```python
from build123d import *

# Parameters (mm, degrees)
SKETCH1_W           = 25
SKETCH1_H           = 40
BOSS_EXTRUDE1_DEPTH = 50
SKETCH2_R           = 4.1
CUT_EXTRUDE1_DEPTH  = 51
SKETCH3_R           = 4.1
CUT_EXTRUDE2_DEPTH  = 41
CUT_EXTRUDE3_DEPTH  = 21
BOSS_EXTRUDE2_DEPTH = 10
BOSS_EXTRUDE3_DEPTH = 10
CHAMFER1_SIZE       = 1
BOSS_EXTRUDE4_DEPTH = 10


with BuildPart() as part:
    # Sketch1 → Boss-Extrude1 (new body)
    with BuildSketch(Plane(origin=(0, 0, 0), x_dir=(1, 0, 0), z_dir=(0, 1, 0))):
        Rectangle(SKETCH1_W, SKETCH1_H)
    extrude(amount=BOSS_EXTRUDE1_DEPTH)

    # Sketch2 → Cut-Extrude1 (cut, through all)
    with BuildSketch(Plane.XZ):
        with Locations((0, -10)):
            Circle(SKETCH2_R)
    extrude(amount=-CUT_EXTRUDE1_DEPTH, mode=Mode.SUBTRACT)

    # Sketch3 → Cut-Extrude2 (cut, through all)
    with BuildSketch(Plane.XY.offset(20)):
        with Locations((0, 17)):
            Circle(SKETCH3_R)
        with Locations((0, 33)):
            Circle(SKETCH3_R)
    extrude(amount=-CUT_EXTRUDE2_DEPTH, mode=Mode.SUBTRACT)

    # Sketch4 → Cut-Extrude3 (cut)
    with BuildSketch(Plane(origin=(0, 0, -20), x_dir=(-1, 0, 0), z_dir=(0, 0, -1))):
        Polygon((-7.5, 17), (-3.75, 10.504809472), (3.75, 10.504809472), (7.5, 17), (3.75, 23.495190528), (-3.75, 23.495190528), align=None)
        Polygon((3.75, 39.495190528), (-3.75, 39.495190528), (-7.5, 33), (-3.75, 26.504809472), (3.75, 26.504809472), (7.5, 33), align=None)
    extrude(amount=-CUT_EXTRUDE3_DEPTH, mode=Mode.SUBTRACT)

    # Sketch5 → Boss-Extrude2 (add)
    with BuildSketch(Plane(origin=(0, 50, 0), x_dir=(1, 0, 0), z_dir=(0, 1, 0))):
        with BuildLine():
            Line((12.5, 5), (20.5, 5))
            Line((20.5, 5), (20.5, 8.1))
            Line((20.5, 8.1), (18.821637353, 8.1))
            ThreePointArc((18.821637353, 8.1), (13.5, 10), (18.821637353, 11.9))
            Line((18.821637353, 11.9), (20.5, 11.9))
            Line((20.5, 11.9), (20.5, 15))
            Line((20.5, 15), (12.5, 15))
            Line((12.5, 15), (12.5, 5))
        make_face()
    extrude(amount=-BOSS_EXTRUDE2_DEPTH)

    # Sketch6 → Boss-Extrude3 (add)
    with BuildSketch(Plane.XY.offset(20)):
        with BuildLine():
            Line((12.5, 12), (20.5, 12))
            Line((20.5, 12), (20.5, 15.1))
            Line((20.5, 15.1), (18.821637353, 15.1))
            ThreePointArc((18.821637353, 15.1), (13.5, 17), (18.821637353, 18.9))
            Line((18.821637353, 18.9), (20.5, 18.9))
            Line((20.5, 18.9), (20.5, 22))
            Line((20.5, 22), (12.5, 22))
            Line((12.5, 22), (12.5, 12))
        make_face()
    extrude(amount=-BOSS_EXTRUDE3_DEPTH)

    # Chamfer1
    chamfer1_edges = [part.edges().sort_by_distance(p)[0] for p in [
        (5.625, 20.247595264, -20),
        (5.625, 13.752404736, -20),
        (0, 10.504809472, -20),
        (-5.625, 13.752404736, -20),
        (-5.625, 20.247595264, -20),
        (0, 23.495190528, -20),
        (-5.625, 36.247595264, -20),
        (0, 39.495190528, -20),
        (5.625, 36.247595264, -20),
        (5.625, 29.752404736, -20),
        (0, 26.504809472, -20),
        (-5.625, 29.752404736, -20),
    ]]
    chamfer(chamfer1_edges, length=CHAMFER1_SIZE)

    # Sketch7 → Boss-Extrude4 (add)
    with BuildSketch(Plane(origin=(0, 50, 0), x_dir=(1, 0, 0), z_dir=(0, 1, 0))):
        Polygon((20.5, 5), (12.5, -20), (12.5, 5), align=None)
    extrude(amount=-BOSS_EXTRUDE4_DEPTH)


solid = part.part
```
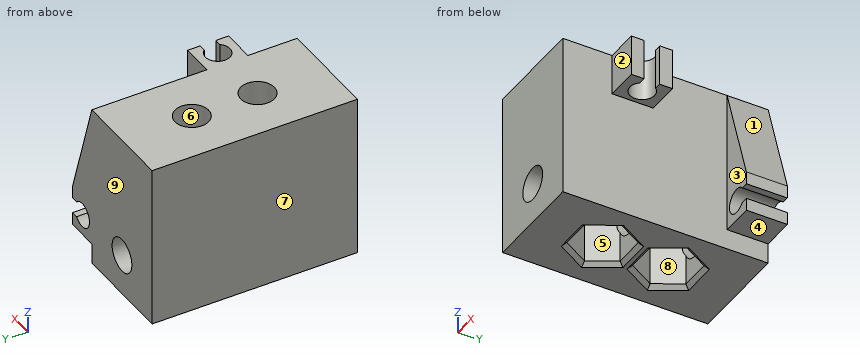
Input: part model. Units: mm. Frame: model coordinates. Face numbers are marked on the shaded views. A direction names the side the tool comes from. Round coordinates to 2 decimals unless told otherwise and drop trailing zeros. Loops run counter-clockwise (first coordinate to the right, second up) from the corner with the lowest first, then second, coordinate; pieces in that order, holes last. Notation, with made-up numbers: (-34, -33) -> (0, -33) arc R6 cw to (0, -26) -> close; hole circle Ø4 at (41.25, -34). An arc over 180 degrees is marked (long way). Write each question's results on one line, items separated by ' | '.
1. First-contact query: P1, Ø2.5, axis at x = 17, z = 16.5, coming from the +Y side; P2, Ø6.5, axis at x = 0.5, y = 15, coming from the -Z side; P3, Ø2.5, axis at x = 18, z = 14, coming from the -Y side; P4, Ø4, axis at x = 17.5, y = 17, coming from the -Z side. Flat tips, straight axial feed; report the tip coordinate or a pass-through.
Geometry results:
P1: y = 22 | P2: z = 1 | P3: y = 12 | P4: through
2. Mould query, pull axis X, two halves, no side actions, for the marked faces 6, 7, 8 and 9. Classes: +X half, -X half, draft (parallel to the pull), parting line (faces both ways), or undercut.
Geometry results:
face 6: undercut | face 7: -X half | face 8: undercut | face 9: draft
3. Section B-B (z = 3). Return loops of the section in (x, y).
Geometry results:
outline: (-12.5, 0) -> (12.5, 0) -> (12.5, 40) -> (17.94, 40) -> (17.94, 50) -> (-12.5, 50) -> close; hole circle Ø8.2 at (0, 17); hole circle Ø8.2 at (0, 33)
4. Ray query, line 1 (Y direction, x = -2, z = -15); line 2 (Y direction, x = 4.5, z = -12); line 3 (X direction, y = 17, z = -11). Return the intervals inside material, ascending. Write a range as from..to.
Geometry results:
line 1: 0..10.5, 23.5..26.5, 39.5..50 | line 2: 0..11.8, 22.2..27.8, 38.2..50 | line 3: -12.5..-7.5, 7.5..12.5
5. Section A-A (x = 16.5). Return loops of the section in (y, z).
Geometry results:
outline: (12, 10) -> (14, 10) -> (14, 20) -> (12, 20) -> close; (20, 10) -> (22, 10) -> (22, 20) -> (20, 20) -> close; (40, -15) -> (50, -15) -> (50, -13) -> (40, -13) -> close; (40, -7) -> (50, -7) -> (50, 7.5) -> (40, 7.5) -> close
6. Section C-C (y = 5.5). Return loops of the section in (x, z), and give its area (3 significant figures).
Geometry results:
outline: (-12.5, -20) -> (12.5, -20) -> (12.5, 20) -> (-12.5, 20) -> close; hole circle Ø8.2 at (0, -10) | area: 947 mm2
7. Set-up query: the marked faces 1, 2, 3, 4 and 5. Return all of +Z, -Z, +X, -X, +Y, -Y with unobstructed straight access to the full face (end or side cutting, diameter ignored); none if empty.
Geometry results:
face 1: +Z, +X, +Y | face 2: +Z, -Z, +X, -Y | face 3: +Z, -Z, +X | face 4: -Z, +X, +Y, -Y | face 5: -Z
8. Section D-D (z = -10). Return loops of the section in (x, y), and give its area (3 significant figures).
Geometry results:
outline: (-12.5, 0) -> (-4.1, 0) -> (-4.1, 11.11) -> (-7.5, 17) -> (-4.1, 22.89) -> (-4.1, 27.11) -> (-7.5, 33) -> (-4.1, 38.89) -> (-4.1, 50) -> (-12.5, 50) -> close; (4.1, 0) -> (12.5, 0) -> (12.5, 40) -> (13.5, 40) -> (13.5, 50) -> (4.1, 50) -> (4.1, 38.89) -> (7.5, 33) -> (4.1, 27.11) -> (4.1, 22.89) -> (7.5, 17) -> (4.1, 11.11) -> close | area: 770 mm2
